CAD build for the part. Positions are in the model's coordinates, mm. Face numbers are marked on the shaded views. A direction names the side the tool comes from. Round coordinates to 2 decimals unless told otherwise and drop trailing zeros. Loops run counter-clockwise (first coordinate to the right, second up) from the corner with the lowest first, then second, coordinate; pieces in that order, holes last. Notation, with made-up numbers: M 45.25,66 L 90.25,66 A35 ccw 90.25,99 Z; hole C -14.5,80 d5. An arc over 180 degrees is marked long. Use a Markdown table: item, result. Add a question column.
(1) Two-plate mould, pull along Y, no slides. Class the marked faces 1, 2, 3 and 4: released by +Y, released by -Y, zero draft, split by the parting line, or undercut.
(2) Band-saw the part on C-C, the plane x = -5. Write the cut outline in (y, z).
(3) Band-saw the part on B-B, the plane z = -9. Write the cut outline in (x, y), and give its area (3 significant figures).
(4) Wall check: L1, parallel to X at y = 27.1, z = 0; L2, parallel to Y at x = 9.7, z = 0; L3, parallel to Y at x = -6.5, z = -2. Give the ranges that are in metal, low to high.
(5) Flat gauge pins, fed straight in: P1, Ø7, axis at x = 5, z = 1.5, coming from the +Y side; P2, Ø2, axis at x = 4, y = -26.5, coming from the -Z side; P3, Ø6, axis at y = -3.5, z = 7, coming from the -X side. Where does each tip first touch, or does it go through?
(6) Which spindle directions (+Z, -Z, +X, -X, +Y, -Y) get a long thin tool onto all of the face, cutting with end or side? Do the marked faces 5 and 6. Say none if no direction does.
(7) Band-saw the part on A-A, the plane y = -21. Write the cut outline in (x, z).
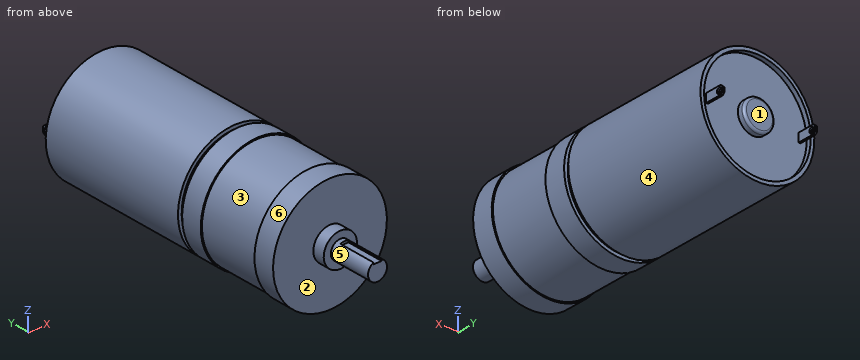
from build123d import *

# Parameters (mm, degrees)
SKETCH2_R           = 12
BOSS_EXTRUDE1_DEPTH = 27.5
SKETCH3_R           = 11.245365849
CUT_EXTRUDE1_DEPTH  = 1
CUT_EXTRUDE2_START  = -23
SKETCH4_R           = 12
SKETCH4_R_2         = 11.226713735
CUT_EXTRUDE2_DEPTH  = 1
CUT_EXTRUDE7_START  = -11
SKETCH5_R           = 12
SKETCH5_R_2         = 11.742388301
CUT_EXTRUDE7_DEPTH  = 6.5
SKETCH6_R           = 3.5
BOSS_EXTRUDE2_DEPTH = 2.5
SKETCH7_R           = 2
BOSS_EXTRUDE3_DEPTH = 9
CUT_EXTRUDE9_DEPTH  = 8
SKETCH9_R           = 3.25
BOSS_EXTRUDE4_DEPTH = 1.5
FILLET2_R           = 0.5
SKETCH10_W          = 0.399131897
SKETCH10_H          = 1.813679108
BOSS_EXTRUDE5_DEPTH = 4
CHAMFER1_SIZE       = 0.4
CHAMFER2_SIZE       = 0.5
SKETCH11_R          = 0.578483289
CUT_EXTRUDE10_DEPTH = 4
CHAMFER3_SIZE       = 0.4
CHAMFER4_SIZE       = 0.4


with BuildPart() as part:
    # Sketch2 → Boss-Extrude1 (new, symmetric)
    with BuildSketch(Plane(origin=(0, 0, 0), x_dir=(1, 0, 0), z_dir=(0, 1, 0))):
        with Locations(Location((0, 0, 0), (0, 0, 270))):
            Circle(SKETCH2_R)
    extrude(amount=BOSS_EXTRUDE1_DEPTH, both=True)

    # Sketch3 → Cut-Extrude1 (cut)
    with BuildSketch(Plane(origin=(0, 27.5, 0), x_dir=(1, 0, 0), z_dir=(0, 1, 0))):
        with Locations(Location((0, 0, 0), (0, 0, 270))):
            Circle(SKETCH3_R)
    extrude(amount=-CUT_EXTRUDE1_DEPTH, mode=Mode.SUBTRACT)

    # Sketch4 → Cut-Extrude2 (cut)
    with BuildSketch(Plane.XZ.offset(27.5).offset(CUT_EXTRUDE2_START)):
        with Locations(Location((0, 0, 0), (0, 0, 270))):
            Circle(SKETCH4_R)
        with Locations(Location((0, 0, 0), (0, 0, 270))):
            Circle(SKETCH4_R_2, mode=Mode.SUBTRACT)
    extrude(amount=CUT_EXTRUDE2_DEPTH, mode=Mode.SUBTRACT)

    # Sketch5 → Cut-Extrude7 (cut, symmetric)
    with BuildSketch(Plane.XZ.offset(27.5).offset(CUT_EXTRUDE7_START)):
        with Locations(Location((0, 0, 0), (0, 0, 270))):
            Circle(SKETCH5_R)
        with Locations(Location((0, 0, 0), (0, 0, 270))):
            Circle(SKETCH5_R_2, mode=Mode.SUBTRACT)
    extrude(amount=CUT_EXTRUDE7_DEPTH, both=True, mode=Mode.SUBTRACT)

    # Sketch6 → Boss-Extrude2 (add)
    with BuildSketch(Plane.XZ.offset(27.5)):
        with Locations(Location((0, 0, 0), (0, 0, 270))):
            Circle(SKETCH6_R)
    extrude(amount=BOSS_EXTRUDE2_DEPTH)

    # Sketch7 → Boss-Extrude3 (add)
    with BuildSketch(Plane.XZ.offset(30)):
        with Locations(Location((0, 0, 0), (0, 0, 270))):
            Circle(SKETCH7_R)
    extrude(amount=BOSS_EXTRUDE3_DEPTH)

    # Sketch8 → Cut-Extrude9 (cut)
    with BuildSketch(Plane.XZ.offset(39)):
        Polygon((0.841690599, 1.659275507), (0.841690599, 2.202635472), (-0.841690599, 2.202635472), (-0.841690599, 1.659275507), (-0.841690599, 1.478155518), (0.841690599, 1.478155518), align=None)
    extrude(amount=-CUT_EXTRUDE9_DEPTH, mode=Mode.SUBTRACT)

    # Sketch9 → Boss-Extrude4 (add)
    with BuildSketch(Plane(origin=(0, 26.5, 0), x_dir=(1, 0, 0), z_dir=(0, 1, 0))):
        with Locations(Location((0, 0, 0), (0, 0, 270))):
            Circle(SKETCH9_R)
    extrude(amount=BOSS_EXTRUDE4_DEPTH)

    # Fillet2
    fillet2_edges = [part.edges().sort_by_distance(p)[0] for p in [
        (0, 28, -3.25),
    ]]
    fillet(fillet2_edges, radius=FILLET2_R)

    # Sketch10 → Boss-Extrude5 (add)
    with BuildSketch(Plane(origin=(0, 26.5, 0), x_dir=(1, 0, 0), z_dir=(0, 1, 0))):
        with Locations((9.751397246, 0)):
            Rectangle(SKETCH10_W, SKETCH10_H)
    boss_extrude5 = extrude(amount=BOSS_EXTRUDE5_DEPTH)

    # Chamfer1
    chamfer1_edges = [part.edges().sort_by_distance(p)[0] for p in [
        (9.751397246, 30.5, -0.906839554),
    ]]
    chamfer(chamfer1_edges, length=CHAMFER1_SIZE)

    # Chamfer2
    chamfer2_edges = [part.edges().sort_by_distance(p)[0] for p in [
        (9.751397246, 30.5, 0.906839554),
    ]]
    chamfer(chamfer2_edges, length=CHAMFER2_SIZE)

    # Sketch11 → Cut-Extrude10 (cut)
    with BuildSketch(Plane(origin=(9.950963194, 0, 0), x_dir=(0, 0, -1), z_dir=(1, 0, 0))):
        with Locations((0, 29.682123993)):
            Circle(SKETCH11_R)
    cut_extrude10 = extrude(amount=-CUT_EXTRUDE10_DEPTH, mode=Mode.SUBTRACT)

    # Mirror1: Boss-Extrude5 across plane
    add(boss_extrude5.mirror(Plane(origin=(0, 0, 0), x_dir=(0, 0, 1), z_dir=(1, 0, 0))))

    # Mirror5: Cut-Extrude10 across plane
    add(cut_extrude10.mirror(Plane(origin=(0, 0, 0), x_dir=(0, 0, 1), z_dir=(1, 0, 0))), mode=Mode.SUBTRACT)

    # Chamfer3
    chamfer3_edges = [part.edges().sort_by_distance(p)[0] for p in [
        (-9.751397246, 30.5, -0.906839554),
    ]]
    chamfer(chamfer3_edges, length=CHAMFER3_SIZE)

    # Chamfer4
    chamfer4_edges = [part.edges().sort_by_distance(p)[0] for p in [
        (-9.751397246, 30.5, 0.906839554),
    ]]
    chamfer(chamfer4_edges, length=CHAMFER4_SIZE)


solid = part.part
Return value:
| question | item | result |
|---|---|---|
| 1 | face 1 | released by +Y |
| 1 | face 2 | released by -Y |
| 1 | face 3 | undercut |
| 1 | face 4 | zero draft |
| 2 | outline | M -27.5,-10.91 L -23,-10.91 L -23,-10.62 L -10,-10.62 L -10,-10.91 L -5.5,-10.91 L -5.5,-10.05 L -4.5,-10.05 L -4.5,-10.91 L 27.5,-10.91 L 27.5,-10.07 L 26.5,-10.07 L 26.5,10.07 L 27.5,10.07 L 27.5,10.91 L -4.5,10.91 L -4.5,10.05 L -5.5,10.05 L -5.5,10.91 L -10,10.91 L -10,10.62 L -23,10.62 L -23,10.91 L -27.5,10.91 Z |
| 3 | outline | M -7.94,-27.5 L 7.94,-27.5 L 7.94,-23 L 7.54,-23 L 7.54,-10 L 7.94,-10 L 7.94,-5.5 L 6.71,-5.5 L 6.71,-4.5 L 7.94,-4.5 L 7.94,27.5 L 6.74,27.5 L 6.74,26.5 L -6.74,26.5 L -6.74,27.5 L -7.94,27.5 L -7.94,-4.5 L -6.71,-4.5 L -6.71,-5.5 L -7.94,-5.5 L -7.94,-10 L -7.54,-10 L -7.54,-23 L -7.94,-23 Z |
| 3 | area | 847 mm^2 |
| 4 | L1 | -12 to -11.25, -9.95 to -9.55, -3.25 to 3.25, 9.55 to 9.95, 11.25 to 12 |
| 4 | L2 | -27.5 to 29.1, 30.26 to 30.5 |
| 4 | L3 | -27.5 to 26.5 |
| 5 | P1 | y = 28 |
| 5 | P2 | z = -11.62 |
| 5 | P3 | x = -11.31 |
| 6 | face 5 | -Y |
| 6 | face 6 | +Y, -Y |
| 7 | outline | C 0,0 d23.48 |
